Geometry check sheet. Reference: the model listing, model coordinates, mm. A direction names the side the tool comes from. Give positions to 0.01 mm unless a question says otherwise; leave off trailing zeros. Write each loop counter-clockwise with the first axis right and the second up, starting at its lowest first coordinate (ties: lowest second). Pieces come first, ordered by that corner, then holes. Notation, with made-up numbers: M 72.25,5 L 84.25,5 A20 ccw 84.25,12 Z; hole C -26.5,72 d1. An arc over 180 degrees is marked long. One line per item, written item: value. Start each with the question number.
1. Cross-section at D-D on z = -9.75. Record the cut outline in (x, y).
2. Cross-section at A-A on x = 0. Record the cut outline in (y, z), then the cut area to 3 significant figures.
3. Gauge pin test, flat ends, axial feed: pin 1 (15 mm diameter, centred on x = -193.5, y = 130, fed in from +Z); pin 2 (8 mm diameter, centred on x = 111, y = -175, fed in from +Z). Record the tip position at first contact, or that the pin passes through.
4. Tool access check on faces 4 (the face through (-128.937, 78.26, -9.392)), 5 (the face through (203, -226, -6.35)). Record the directions out of +Z, -Z, +X, -X, +Y, -Y that give a thin tool (end or side, any length) a straight path to the whole face; none if there is none.
5. Scan lines: line 1 (X direction, y = 131, z = -2.25); line 2 (Y direction, x = 214, z = -1); line 3 (Y direction, x = 0, z = -10.75). Record each from-to range of solid material in increasing order.
6. Cross-section at B-B on y = 0. Record the cut outline in (x, z), then the cut area to 3 significant figures.
7. Release check for a two-part mould opening along X. For faces 1 (the face through (-3, 189.588, -9)), 2 (the face through (-204, -226, -6.35)), 3 (the face through (246.757, 181.95, -9.658)) record: pulls with the +X half, pulls with the -X half, needs draft (parallel to the pull), parting line crosses it, or undercut.
8. Cross-section at C-C on x = 152.4. Record the cut outline in (y, z), then the cut area to 3 significant figures.
from build123d import *

# Parameters (mm, degrees)
F0_W     = 508
F0_H     = 467.164543
F0_W_2   = 50.8
F0_H_2   = 50.8
F0_R     = 25.4
F0_R_2   = 87.988181
F1_DEPTH = 19.05
F2_R     = 25.4
F3_DEPTH = 6.35
F4_DEPTH = 19.051


with BuildPart() as f1:
    # F0 (on Top) → F1 (new body)
    with BuildSketch(Plane.XY):
        with Locations((0, -43.99409)):
            Rectangle(F0_W, F0_H)
        with Locations((-203.2, -226.776362)):
            Rectangle(F0_W_2, F0_H_2, mode=Mode.SUBTRACT)
        with Locations((0, -175.976362)):
            Circle(F0_R, mode=Mode.SUBTRACT)
        with Locations((203.2, -226.776362)):
            Rectangle(F0_W_2, F0_H_2, mode=Mode.SUBTRACT)
        with Locations((-152.4, 87.988181)):
            Circle(F0_R, mode=Mode.SUBTRACT)
        with Locations((-203.2, 138.788181)):
            Rectangle(F0_W_2, F0_H_2, mode=Mode.SUBTRACT)
        Circle(F0_R_2, mode=Mode.SUBTRACT)
        with Locations((152.4, 87.988181)):
            Circle(F0_R, mode=Mode.SUBTRACT)
        with Locations((203.2, 138.788181)):
            Rectangle(F0_W_2, F0_H_2, mode=Mode.SUBTRACT)
        with Locations((-203.2, 138.788181)):
            Rectangle(F0_W_2, F0_H_2)
        with Locations((-203.2, -226.776362)):
            Rectangle(F0_W_2, F0_H_2)
        with Locations((203.2, -226.776362)):
            Rectangle(F0_W_2, F0_H_2)
        with Locations((203.2, 138.788181)):
            Rectangle(F0_W_2, F0_H_2)
        with Locations((-152.4, 87.988181)):
            Circle(F0_R)
        with Locations((152.4, 87.988181)):
            Circle(F0_R)
        with Locations((0, -175.976362)):
            Circle(F0_R)
    extrude(amount=-F1_DEPTH)

    # F2
    f2_edges = [f1.edges().sort_by_distance(p)[0] for p in [
        (-254, 189.588181, -9.525),
        (254, 189.588181, -9.525),
        (-254, -277.576362, -9.525),
        (254, -277.576362, -9.525),
    ]]
    fillet(f2_edges, radius=F2_R)

    # F0 (on Top) → F3 (cut)
    with BuildSketch(Plane.XY):
        with Locations((-203.2, -226.776362)):
            Rectangle(F0_W_2, F0_H_2)
        with Locations((-203.2, 138.788181)):
            Rectangle(F0_W_2, F0_H_2)
        with Locations((203.2, -226.776362)):
            Rectangle(F0_W_2, F0_H_2)
        with Locations((203.2, 138.788181)):
            Rectangle(F0_W_2, F0_H_2)
    extrude(amount=-F3_DEPTH, mode=Mode.SUBTRACT)

    # F0 (on Top) → F4 (cut, through all)
    with BuildSketch(Plane.XY):
        with Locations((-152.4, 87.988181)):
            Circle(F0_R)
        with Locations((0, -175.976362)):
            Circle(F0_R)
        with Locations((152.4, 87.988181)):
            Circle(F0_R)
    extrude(amount=-F4_DEPTH, mode=Mode.SUBTRACT)


solid = f1.part
Report:
1. outline: M -254,-252.18 A25.4 ccw -228.6,-277.58 L 228.6,-277.58 A25.4 ccw 254,-252.18 L 254,164.19 A25.4 ccw 228.6,189.59 L -228.6,189.59 A25.4 ccw -254,164.19 Z; hole C -152.4,87.99 d50.8; hole C 0,0 d175.98; hole C 0,-175.98 d50.8; hole C 152.4,87.99 d50.8
2. outline: M -277.58,-19.05 L -201.38,-19.05 L -201.38,0 L -277.58,0 Z; M -150.58,-19.05 L -87.99,-19.05 L -87.99,0 L -150.58,0 Z; M 87.99,-19.05 L 189.59,-19.05 L 189.59,0 L 87.99,0 Z
2. area: 4,580 mm^2
3. pin 1: stops at z = -6.35
3. pin 2: stops at z = 0
4. face 4: +Z, -Z
4. face 5: +Z
5. line 1: x = -254 to -228.6, -177.8 to 177.8, 228.6 to 254
5. line 2: y = -277.58 to -252.18, -201.38 to 113.39, 164.19 to 189.59
5. line 3: y = -277.58 to -201.38, -150.58 to -87.99, 87.99 to 189.59
6. outline: M -254,-19.05 L -87.99,-19.05 L -87.99,0 L -254,0 Z; M 87.99,-19.05 L 254,-19.05 L 254,0 L 87.99,0 Z
6. area: 6,330 mm^2
7. face 1: needs draft
7. face 2: undercut
7. face 3: pulls with the +X half
8. outline: M -277.58,-19.05 L 62.59,-19.05 L 62.59,0 L -277.58,0 Z; M 113.39,-19.05 L 189.59,-19.05 L 189.59,0 L 113.39,0 Z
8. area: 7,930 mm^2
